For this review, take the finished solid that the model builds, in its own axes (mm). Face numbers are marked on the shaded views. A direction names the side the tool comes from. Coordinates: 2 decimals unless noted, no trailing zeros. Write each loop counter-clockwise with the first axis right and the second up, starting at its lowest first coordinate (ties: lowest second). Pieces come first, ordered by that corner, then holes. Notation, with made-up numbers: M 9.5,74 L 30.5,74 A21 cw 30.5,81 Z; hole C -40,86.5 d11. An arc over 180 degrees is marked long. Return JSON: item names as keys, results as strings.
```python
from build123d import *

# Parameters (mm, degrees)
SKETCH1_R           = 27.5
SKETCH1_R_2         = 15
BOSS_EXTRUDE1_DEPTH = 18
BOSS_EXTRUDE2_DEPTH = 6
SKETCH1_4_R         = 20
SKETCH1_4_R_2       = 9
BOSS_EXTRUDE3_DEPTH = 18
SKETCH2_R           = 20
SKETCH2_R_2         = 9
CUT_EXTRUDE1_DEPTH  = 12
SKETCH1_5_W         = 140
SKETCH1_5_H         = 18
BOSS_EXTRUDE4_DEPTH = 79
CUT_EXTRUDE2_REACH  = 171.486
SKETCH4_R           = 8
CUT_EXTRUDE3_REACH  = 201.412
SKETCH5_W           = 3
SKETCH5_H           = 49
SKETCH1_6_W         = 140
SKETCH1_6_H         = 18
BOSS_EXTRUDE5_DEPTH = 6


with BuildPart() as part:
    # Sketch1 → Boss-Extrude1 (new, symmetric)
    with BuildSketch(Plane(origin=(0, 0, 0), x_dir=(1, 0, 0), z_dir=(0, 1, 0))):
        with Locations(Location((0, 0, 0), (0, 0, 270))):
            Circle(SKETCH1_R)
        with Locations(Location((0, 0, 0), (0, 0, 270))):
            Circle(SKETCH1_R_2, mode=Mode.SUBTRACT)
    extrude(amount=BOSS_EXTRUDE1_DEPTH, both=True)

    # Sketch1_3 → Boss-Extrude2 (add, symmetric)
    with BuildSketch(Plane(origin=(0, 0, 0), x_dir=(1, 0, 0), z_dir=(0, 1, 0))):
        with BuildLine():
            Line((-78.919837001, -62), (-78.919837001, -100))
            Line((-78.919837001, -100), (61.080162999, -100))
            Line((61.080162999, -100), (27.5, 0))
            ThreePointArc((27.5, 0), (4.798237479, -27.078163104), (-25.82559397, -9.449269605))
            ThreePointArc((-25.82559397, -9.449269605), (-30.4703787, -34.480836347), (-54.645867965, -42.462006534))
            ThreePointArc((-54.645867965, -42.462006534), (-43.339731406, -49.45965273), (-38.919837001, -62))
            ThreePointArc((-38.919837001, -62), (-58.919837001, -82), (-78.919837001, -62))
        make_face()
    extrude(amount=BOSS_EXTRUDE2_DEPTH, both=True)

    # Sketch1_4 → Boss-Extrude3 (add, symmetric)
    with BuildSketch(Plane(origin=(0, 0, 0), x_dir=(1, 0, 0), z_dir=(0, 1, 0))):
        with Locations(Location((-58.919837001, -62, 0), (0, 0, 270))):
            Circle(SKETCH1_4_R)
        with Locations(Location((-58.919837001, -62, 0), (0, 0, 270))):
            Circle(SKETCH1_4_R_2, mode=Mode.SUBTRACT)
    extrude(amount=BOSS_EXTRUDE3_DEPTH, both=True)

    # Sketch2 → Cut-Extrude1 (cut)
    with BuildSketch(Plane.XZ.offset(18)):
        with Locations(Location((-58.919837001, 62, 0), (0, 0, 282.339179535))):
            Circle(SKETCH2_R)
        with Locations(Location((-58.919837001, 62, 0), (0, 0, 270))):
            Circle(SKETCH2_R_2, mode=Mode.SUBTRACT)
    extrude(amount=-CUT_EXTRUDE1_DEPTH, mode=Mode.SUBTRACT)

    # Sketch1_5 → Boss-Extrude4 (add)
    with BuildSketch(Plane(origin=(0, 0, 0), x_dir=(1, 0, 0), z_dir=(0, 1, 0))):
        with Locations((-8.919837001, -109)):
            Rectangle(SKETCH1_5_W, SKETCH1_5_H)
    extrude(amount=BOSS_EXTRUDE4_DEPTH)

    # Sketch4 → Cut-Extrude2 (cut, up to next)
    with BuildSketch(Plane(origin=(0, 0, 100), x_dir=(-1, 0, 0), z_dir=(0, 0, -1)), mode=Mode.PRIVATE) as cut_extrude2_sk1:
        with Locations((-26.080162999, 49)):
            Circle(SKETCH4_R)
    cut_extrude2_tool1 = extrude(cut_extrude2_sk1.sketch, amount=-CUT_EXTRUDE2_REACH, mode=Mode.PRIVATE) & part.part
    # Sketch4 → Cut-Extrude2 (cut, up to next)
    with BuildSketch(Plane(origin=(0, 0, 100), x_dir=(-1, 0, 0), z_dir=(0, 0, -1)), mode=Mode.PRIVATE) as cut_extrude2_sk2:
        with Locations((43.919837001, 49)):
            Circle(SKETCH4_R)
    cut_extrude2_tool2 = extrude(cut_extrude2_sk2.sketch, amount=-CUT_EXTRUDE2_REACH, mode=Mode.PRIVATE) & part.part
    add(cut_extrude2_tool1.solids().sort_by_distance((26.080163, 49, 100))[0], mode=Mode.SUBTRACT)
    add(cut_extrude2_tool2.solids().sort_by_distance((-43.919837, 49, 100))[0], mode=Mode.SUBTRACT)

    # Sketch5 → Cut-Extrude3 (cut, up to next)
    with BuildSketch(Plane.ZY.offset(78.919837001), mode=Mode.PRIVATE) as cut_extrude3_sk1:
        with Locations((116.5, 36.5)):
            Rectangle(SKETCH5_W, SKETCH5_H)
    cut_extrude3_tool1 = extrude(cut_extrude3_sk1.sketch, amount=-CUT_EXTRUDE3_REACH, mode=Mode.PRIVATE) & part.part
    add(cut_extrude3_tool1.solids().sort_by_distance((-78.919837, 36.5, 116.5))[0], mode=Mode.SUBTRACT)

    # Sketch1_6 → Boss-Extrude5 (add)
    with BuildSketch(Plane(origin=(0, 0, 0), x_dir=(1, 0, 0), z_dir=(0, 1, 0))):
        with Locations((-8.919837001, -109)):
            Rectangle(SKETCH1_6_W, SKETCH1_6_H)
    extrude(amount=-BOSS_EXTRUDE5_DEPTH)


solid = part.part
```
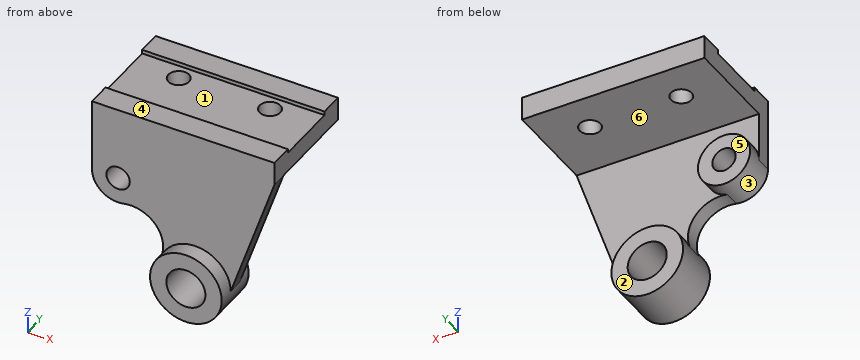
1. We need section D-D (z = 58). State the section outline as (x, y) points, plus the area to 3 significant figures.
Checks:
{"outline": "M -78.52,-6 L -66.98,-6 L -66.98,18 L -78.52,18 Z; M -50.86,-6 L 46.98,-6 L 46.98,6 L -39.32,6 L -39.32,18 L -50.86,18 Z", "area": "1,590 mm2"}
2. Draft analysis for pull direction Z (two halves, no side actions). For the marked faces 4, 5 and 6, state which applies: +Z half, -Z half, draft (parallel to the pull), parting line (faces both ways), or undercut.
Checks:
{"face 4": "+Z half", "face 5": "draft", "face 6": "undercut"}
3. Wall thickness on L1, parallel to X at y = 52.5, z = 101.5; L2, parallel to X at y = 4, z = 0; L3, parallel to Z at x = 21.5, y = 72: over which ranges is each line inside the solid? List them lowest first. Write a range as from..to.
Checks:
{"L1": "-78.92..-51.11, -36.73..18.89, 33.27..61.08", "L2": "-27.5..-15, 15..27.5", "L3": "100..118"}
4. Clearance check with flat-ended pins moving along their axes: pin 1 Ø2 at (x, z) = (17.5, 71.5) entering from +Y; pin 2 Ø10 at (x, z) = (6.5, -1) entering from +Y; pin 3 Ø10 at (y, z) = (19, -7) entering from +X; pin 4 Ø22 at (x, y) = (-2.5, 39.5) entering from -Z. State where each tip first meets the part, or that it passes through.
Checks:
{"pin 1": "y = 6", "pin 2": "through", "pin 3": "x = 27.42", "pin 4": "z = 100"}
5. We need section B-B (x = 0). State the section outline as (y, z) points, plus the area to 3 significant figures.
Checks:
{"outline": "M -18,-27.5 L 18,-27.5 L 18,-15 L -18,-15 Z; M -18,15 L 18,15 L 18,27.5 L 6,27.5 L 6,100 L 79,100 L 79,118 L 61,118 L 61,115 L 12,115 L 12,118 L -6,118 L -6,27.5 L -18,27.5 Z", "area": "3,150 mm2"}
6. We need section C-C (y = 49). State the section outline as (x, z) points.
Checks:
{"outline": "M -78.92,100 L -51.92,100 L -51.92,115 L -78.92,115 Z; M -35.92,100 L 18.08,100 L 18.08,115 L -35.92,115 Z; M 34.08,100 L 61.08,100 L 61.08,115 L 34.08,115 Z"}
7. For the marked faces 1, 2 and 3, list the 3-axis set-ups (+Z, -Z, +X, -X, +Y, -Y) from which the entire face can be reached by the end or side of a thin tool; tool diameter is ignored.
Checks:
{"face 1": "+Z, +X, -X", "face 2": "-Z, +X, -X, +Y", "face 3": "+Y"}
8. We need section A-A (y = 15). State the section outline as (x, z) points, plus the area to 3 significant figures.
Checks:
{"outline": "C -58.92,62 d40; M -78.92,100 L 61.08,100 L 61.08,115 L -78.92,115 Z; C 0,0 d55; hole C -58.92,62 d18; hole C 0,0 d30", "area": "4,770 mm2"}
